Geometry check sheet. Reference: the model listing, model coordinates, mm. A direction names the side the tool comes from. Coordinates: 2 decimals unless noted, no trailing zeros. Loops run counter-clockwise (first coordinate to the right, second up) from the corner with the lowest first, then second, coordinate; pieces in that order, holes last.
Autodesk Inventor part; units mm, degrees
ref_plane "Work Plane1" through (-47.5, 5, 60) normal (1, 0, 0) x (0, 0, -1)
ref_plane "YZ Plane" through (0, 0, 0) normal (1, 0, 0) x (0, 1, 0)
ref_plane "XZ Plane" through (0, 0, 0) normal (0, 1, 0) x (-1, 0, 0)
sketch "Sketch1" plane through (0, 0, 0) normal (0, 1, 0) x (-1, 0, 0)
  line L0 (0, 0) -> (95, 0)
  line L1 (95, 0) -> (95, 65)
  line L2 (95, 65) -> (0, 65)
  line L3 (0, 65) -> (0, 0)
extrude "Extrusion1" add sketch "Sketch1" along normal blind 20
sketch "Sketch2" plane through (0, 20, 0) normal (0, 1, 0) x (1, 0, 0)
  line L0 (-5, -5) -> (-90, -5)
  line L1 (-90, -5) -> (-90, -60)
  line L2 (-90, -60) -> (-5, -60)
  line L3 (-5, -60) -> (-5, -5)
extrude "Extrusion2" cut sketch "Sketch2" against normal blind 15
sketch "Sketch5" plane through (-90, 20, 60) normal (1, 0, 0) x (0, 0, -1)
  line L0 (0, -15) -> (55, -15)
  line L1 (21, -4) -> (39, -4)
  line L2 (39, -4) -> (39, 10)
  line L3 (39, 10) -> (21, 10)
  line L4 (21, 10) -> (21, -4)
  point P0 (60, -20)
  point P1 (60, 0)
  dimension "d12" = 18
  dimension "d13" = 14
  dimension "d15" = 21
  dimension "d16" = 11
extrude "Extrusion3" add sketch "Sketch5" along normal blind 2
ref_plane "Work Plane1" through (-47.5, 5, 60) normal (1, 0, 0) x (0, 0, -1)
mirror "Mirror1" about plane through (-47.5, 5, 60) normal (1, 0, 0) of "Extrusion3"
sketch "Sketch7" plane through (-5, 20, 21) normal (1, 0, 0) x (0, 0, -1)
  line L0 (0, 10) -> (-18, 10)
  line L1 (-18, 10) -> (-18, 0)
  point P0 (21, -20)
  point P1 (-9, 7.5)
  dimension "d19" = 9
  dimension "d20" = 2.5
hole "Hole2" at (-5, 27.5, 30) direction (-1, 0, 0) diameter 3.25 end through all
properties part number "RESONATORCHAMBER"
1) Mould release check, pull along Z, two halves, no side actions. Record for faces 4 (the flat face through (-6, 30, 30)), 5 (the flat face through (-7, 23, 30)), 6 (the flat face through (-47, 10, 0)): +Z half, -Z half, draft (parallel to the pull), parting line (faces both ways), or undercut.
Data:
face 4: draft
face 5: undercut
face 6: -Z half
2) Access from +Z, -Z, +X, -X, +Y, -Y to the whole of each face (thin tool, end or side, straight path). Record for faces 1 (the flat face through (-90, 25, 30)), 2 (the flat face through (-89, 23, 21)), 3 (the flat face through (-89, 16, 30)).
Data:
face 1: +Z, -Z, -X, +Y
face 2: +Y
face 3: none
3) Section check D-D on z = 13.5. Record the cut outline in (x, y).
Data:
outline: (-95, 0) - (0, 0) - (0, 20) - (-5, 20) - (-5, 5) - (-90, 5) - (-90, 20) - (-95, 20) - close
4) Section check C-C on x = -13. Record the cut outline in (y, z), and give its area (3 significant figures).
Data:
outline: (0, 0) - (20, 0) - (20, 5) - (5, 5) - (5, 60) - (20, 60) - (20, 65) - (0, 65) - close
area: 475 mm2
5) Section check A-A on z = 30. Record the cut outline in (x, y) (3 decimals), and give its area (3 significant figures).
Data:
outline: (-95, 0) - (0, 0) - (0, 20) - (-5, 20) - (-5, 25.875) - (-7, 25.875) - (-7, 16) - (-5, 16) - (-5, 5) - (-90, 5) - (-90, 16) - (-88, 16) - (-88, 25.875) - (-90, 25.875) - (-90, 20) - (-95, 20) - close; (-90, 29.125) - (-88, 29.125) - (-88, 30) - (-90, 30) - close; (-7, 29.125) - (-5, 29.125) - (-5, 30) - (-7, 30) - close
area: 668 mm2
6) Depth check by flat-ended pin: pin 1 (6 mm diameter, centred on y = 23.5, z = 17, fed in from +X); pin 2 (4 mm diameter, centred on y = 27.5, z = 30, fed in from +X); pin 3 (1 mm diameter, centred on x = -6, y = 22, fed in from +Z); pin 4 (5 mm diameter, centred on y = 23, z = 26, fed in from -X). Enter the tip coordinate at first touch or a pass-through.
Data:
pin 1: passes through
pin 2: stops at x = -5
pin 3: stops at z = 39
pin 4: stops at x = -90
7) Material ranges on probe 1 along Y at (x, z) = (-89.3, 30) (3 decimals); probe 2 along Z at (x, y) = (-71, 19); probe 3 along Z at (x, y) = (-5.5, 27.5) (3 decimals), recorded low to high.
Data:
probe 1: y = 0 to 5, 16 to 25.875, 29.125 to 30
probe 2: z = 0 to 5, 60 to 65
probe 3: z = 21 to 28.375, 31.625 to 39
8) Section check B-B on y = 8.5. Record the cut outline in (x, z).
Data:
outline: (-95, 0) - (0, 0) - (0, 65) - (-95, 65) - close; hole (-90, 5) - (-5, 5) - (-5, 60) - (-90, 60) - close
